```python
from build123d import *

# Parameters (mm, degrees)
SKETCH1_W                    = 119
SKETCH1_H                    = 89
BOSS_EXTRUDE2_DEPTH          = 3
SKETCH3_W                    = 89
SKETCH3_H                    = 89
SKETCH3_W_2                  = 85
SKETCH3_H_2                  = 85
BOSS_EXTRUDE3_DEPTH          = 25
SKETCH4_W                    = 87
SKETCH4_H                    = 87
CUT_EXTRUDE1_DEPTH           = 2
SKETCH6_W                    = 8
SKETCH6_H                    = 8
BOSS_EXTRUDE4_DEPTH          = 2
SKETCH7_R                    = 2
CUT_EXTRUDE2_DEPTH           = 4.8
SKETCH8_W                    = 9
SKETCH8_H                    = 11
SKETCH8_W_2                  = 12
SKETCH8_W_3                  = 13
SKETCH8_H_2                  = 12
CUT_EXTRUDE3_DEPTH           = 2
SKETCH9_W                    = 13
SKETCH9_H                    = 11
CUT_EXTRUDE4_DEPTH           = 2
SKETCH10_R                   = 1.6
CUT_EXTRUDE5_DEPTH           = 3
SKETCH11_W                   = 7
SKETCH11_H                   = 25
CUT_EXTRUDE6_DEPTH           = 1
FILLET2_R                    = 2
CSK_FOR_M3_SFHCS1_AT_2_COUNT = 2
CSK_FOR_M3_SFHCS1_AT_2_PITCH = 69
CSK_FOR_M3_SFHCS1_AT_3_COUNT = 2
CSK_FOR_M3_SFHCS1_AT_3_PITCH = 124.807852317
CSK_FOR_M3_SFHCS1_AT_4_COUNT = 2
CSK_FOR_M3_SFHCS1_AT_4_PITCH = 104


with BuildPart() as part:
    # Sketch1 → Boss-Extrude2 (new body)
    with BuildSketch(Plane(origin=(0, 0, 0), x_dir=(1, 0, 0), z_dir=(0, 1, 0))):
        Rectangle(SKETCH1_W, SKETCH1_H)
    extrude(amount=BOSS_EXTRUDE2_DEPTH)

    # Sketch3 → Boss-Extrude3 (add)
    with BuildSketch(Plane(origin=(0, 3, 0), x_dir=(1, 0, 0), z_dir=(0, 1, 0))):
        Rectangle(SKETCH3_W, SKETCH3_H)
        Rectangle(SKETCH3_W_2, SKETCH3_H_2, mode=Mode.SUBTRACT)
    extrude(amount=BOSS_EXTRUDE3_DEPTH)

    # Sketch4 → Cut-Extrude1 (cut)
    with BuildSketch(Plane(origin=(0, 28, 0), x_dir=(1, 0, 0), z_dir=(0, 1, 0))):
        Rectangle(SKETCH4_W, SKETCH4_H)
    extrude(amount=-CUT_EXTRUDE1_DEPTH, mode=Mode.SUBTRACT)

    # Sketch6 → Boss-Extrude4 (add)
    with BuildSketch(Plane(origin=(0, 3, 0), x_dir=(1, 0, 0), z_dir=(0, 1, 0))):
        with Locations((-38.5, -38.5)):
            Rectangle(SKETCH6_W, SKETCH6_H)
        with Locations((-38.5, 38.5)):
            Rectangle(SKETCH6_W, SKETCH6_H)
        with Locations((38.5, 38.5)):
            Rectangle(SKETCH6_W, SKETCH6_H)
        with Locations((38.5, -38.5)):
            Rectangle(SKETCH6_W, SKETCH6_H)
    extrude(amount=BOSS_EXTRUDE4_DEPTH)

    # Sketch7 → Cut-Extrude2 (cut)
    with BuildSketch(Plane(origin=(0, 5, 0), x_dir=(1, 0, 0), z_dir=(0, 1, 0))):
        with Locations((-38.5, 38.5)):
            Circle(SKETCH7_R)
        with Locations((38.5, 38.5)):
            Circle(SKETCH7_R)
        with Locations((-38.5, -38.5)):
            Circle(SKETCH7_R)
        with Locations((38.5, -38.5)):
            Circle(SKETCH7_R)
    extrude(amount=-CUT_EXTRUDE2_DEPTH, mode=Mode.SUBTRACT)

    # Sketch8 → Cut-Extrude3 (cut)
    with BuildSketch(Plane(origin=(-42.5, 0, 0), x_dir=(0, 0, -1), z_dir=(1, 0, 0))):
        with Locations((16.4, 13.5)):
            Rectangle(SKETCH8_W, SKETCH8_H)
        with Locations((1.4, 13.5)):
            Rectangle(SKETCH8_W_2, SKETCH8_H)
        with Locations((-14.5, 14)):
            Rectangle(SKETCH8_W_3, SKETCH8_H_2)
    extrude(amount=-CUT_EXTRUDE3_DEPTH, mode=Mode.SUBTRACT)

    # Sketch9 → Cut-Extrude4 (cut)
    with BuildSketch(Plane(origin=(0, 0, 42.5), x_dir=(-1, 0, 0), z_dir=(0, 0, -1))):
        with Locations((8.5, 13.5)):
            Rectangle(SKETCH9_W, SKETCH9_H)
        with Locations((25.5, 13.5)):
            Rectangle(SKETCH9_W, SKETCH9_H)
        with Locations((-8.5, 13.5)):
            Rectangle(SKETCH9_W, SKETCH9_H)
        with Locations((-25.5, 13.5)):
            Rectangle(SKETCH9_W, SKETCH9_H)
    extrude(amount=-CUT_EXTRUDE4_DEPTH, mode=Mode.SUBTRACT)

    # Sketch10 → Cut-Extrude5 (cut)
    with BuildSketch(Plane(origin=(0, 3, 0), x_dir=(1, 0, 0), z_dir=(0, 1, 0))):
        with Locations((-52, 34.5)):
            Circle(SKETCH10_R)
        with Locations((-52, -34.5)):
            Circle(SKETCH10_R)
        with Locations((52, 34.5)):
            Circle(SKETCH10_R)
        with Locations((52, -34.5)):
            Circle(SKETCH10_R)
    extrude(amount=-CUT_EXTRUDE5_DEPTH, mode=Mode.SUBTRACT)

    # Sketch11 → Cut-Extrude6 (cut)
    with BuildSketch(Plane(origin=(0, 3, 0), x_dir=(1, 0, 0), z_dir=(0, 1, 0))):
        with Locations((52, -14.77145541)):
            Rectangle(SKETCH11_W, SKETCH11_H)
    extrude(amount=-CUT_EXTRUDE6_DEPTH, mode=Mode.SUBTRACT)

    # Fillet2
    fillet2_edges = [part.edges().sort_by_distance(p)[0] for p in [
        (59.5, 3, 0),
        (52, 3, 44.5),
        (-52, 3, -44.5),
        (52, 3, -44.5),
        (-44.5, 3, 0),
        (-44.5, 15.5, -44.5),
        (-44.5, 15.5, 44.5),
        (44.5, 3, 0),
        (44.5, 15.5, 44.5),
        (44.5, 15.5, -44.5),
        (-59.5, 3, 0),
        (-59.5, 1.5, -44.5),
        (59.5, 1.5, -44.5),
        (59.5, 1.5, 44.5),
        (-59.5, 1.5, 44.5),
        (-52, 3, 44.5),
    ]]
    fillet(fillet2_edges, radius=FILLET2_R)

    # Sketch13 → CSK for M3 SFHCS1 (revolve, cut)
    with BuildSketch(Plane(origin=(52, 3, -34.5), x_dir=(0, 0, 1), z_dir=(1, 0, 0))):
        Polygon((0, 0), (0, 3), (1.7, 3), (1.7, 1.66), (3.36, 0), align=None)
    csk_for_m3_sfhcs1 = revolve(axis=Axis((52, 9.35, -34.5), (0, -1, 0)), mode=Mode.SUBTRACT)

    # CSK for M3 SFHCS1 at 2: CSK for M3 SFHCS1 ×2
    with Locations(*[(0, 0, i * CSK_FOR_M3_SFHCS1_AT_2_PITCH) for i in range(1, CSK_FOR_M3_SFHCS1_AT_2_COUNT)]):
        add(csk_for_m3_sfhcs1, mode=Mode.SUBTRACT)

    # CSK for M3 SFHCS1 at 3: CSK for M3 SFHCS1 ×2
    with Locations(*[Vector(-0.833280904, 0, 0.552849831) * (i * CSK_FOR_M3_SFHCS1_AT_3_PITCH) for i in range(1, CSK_FOR_M3_SFHCS1_AT_3_COUNT)]):
        add(csk_for_m3_sfhcs1, mode=Mode.SUBTRACT)

    # CSK for M3 SFHCS1 at 4: CSK for M3 SFHCS1 ×2
    with Locations(*[(-i * CSK_FOR_M3_SFHCS1_AT_4_PITCH, 0, 0) for i in range(1, CSK_FOR_M3_SFHCS1_AT_4_COUNT)]):
        add(csk_for_m3_sfhcs1, mode=Mode.SUBTRACT)


solid = part.part
```
Geometry check sheet. Reference: the model listing, model coordinates, mm. A direction names the side the tool comes from. Give positions to 0.01 mm unless a question says otherwise; leave off trailing zeros. Order: outer loops, then holes, each group sorted by start corner. A loop starts at its lowest first (then second) coordinate and runs counter-clockwise, first axis right, second up. Notation, with made-up numbers: (8, 75) - (59, 75) arc R37 ccw to (59, 112) - close; hole circle Ø2 at (-28.75, -37.5). An arc over 180 degrees is marked (long way). Write item = value, one per line. Start each with the question number.
1) Section check A-A (z = 17). Enter the section's corners in (x, y).
2) Section check D-D (y = 16.75). Count the separate pieces of the cut face and the enclosed holes in it, then the cut area to 3 significant figures.
3) Gauge pin test, flat ends, axial feed: pin 1 Ø12 at (y, z) = (25, 6.5) entering from +X; pin 2 Ø4 at (y, z) = (16, 20.5) entering from -X; pin 3 Ø1 at (x, y) = (-44, 13.5) entering from -Z. Record the tip position at first contact, or that the pin passes through.
4) Section check B-B (x = 52). Enter the section's corners in (y, z).
5) Draft check along X on faces 1 (the cylindrical face through (-38.934, 2.634, 40.452)), 2 (the flat face through (52, 3, -1)), 3 (the flat face through (44.5, 16, 1)). Enter one of: released by +X, released by -X, zero draft, split by the parting line, or undercut.
6) Scan lines: L1, parallel to Z at x = 52, y = 0.9; L2, parallel to Z at x = -38.5, y = 2.7; L3, parallel to X at y = 0.6, z = -34.5. Record each from-to range of solid material in increasing order.
7) Access from +Z, -Z, +X, -X, +Y, -Y to the whole of each face (thin tool, end or side, straight path). Record for faces 4 (the flat face through (-1, 14, -44.5)), 5 (the flat face through (-52, 3, -1)), 6 (the flat face through (36.7, 5, 36.7)).
8) Section check C-C (x = -38.5). Enter the section's corners in (y, z).
Geometry check:
q1.outline = (-59.5, 0) - (59.5, 0) - (59.5, 1) arc R2 ccw to (57.5, 3) - (55.5, 3) - (55.5, 2) - (48.5, 2) - (48.5, 3) - (46.5, 3) arc R2 cw to (44.5, 5) - (44.5, 28) - (43.5, 28) - (43.5, 26) - (42.5, 26) - (42.5, 3) - (-42.5, 3) - (-42.5, 8) - (-44.5, 8) - (-44.5, 5) arc R2 cw to (-46.5, 3) - (-57.5, 3) arc R2 ccw to (-59.5, 1) - close; (-44.5, 20) - (-42.5, 20) - (-42.5, 26) - (-43.5, 26) - (-43.5, 28) - (-44.5, 28) - close
q2.separate_pieces = 7
q2.enclosed_holes = 0
q2.area = 521 mm2
q3.pin_1 = 44.5
q3.pin_2 = -44.5
q3.pin_3 = -44.23
q4.outline = (0, -44.5) - (1, -44.5) arc R2 ccw to (3, -42.5) - (3, -37.86) - (1.34, -36.2) - (0, -36.2) - close; (0, -32.8) - (1.34, -32.8) - (3, -31.14) - (3, 2.27) - (2, 2.27) - (2, 27.27) - (3, 27.27) - (3, 31.14) - (1.34, 32.8) - (0, 32.8) - close; (0, 36.2) - (1.34, 36.2) - (3, 37.86) - (3, 42.5) arc R2 ccw to (1, 44.5) - (0, 44.5) - close
q5.face_1 = undercut
q5.face_2 = zero draft
q5.face_3 = released by +X
q6.L1 = -44.5 to -36.2, -32.8 to 32.8, 36.2 to 44.5
q6.L2 = -44.5 to -40.5, -36.5 to 36.5, 40.5 to 44.5
q6.L3 = -59.5 to -53.7, -50.3 to 50.3, 53.7 to 59.5
q7.face_4 = -Z, +X, -X, +Y, -Y
q7.face_5 = +Z, -Z, -X, +Y
q7.face_6 = +Y
q8.outline = (0, -44.5) - (28, -44.5) - (28, -43.5) - (26, -43.5) - (26, -42.5) - (5, -42.5) - (5, -40.5) - (0.2, -40.5) - (0.2, -36.5) - (5, -36.5) - (5, -34.5) - (3, -34.5) - (3, 34.5) - (5, 34.5) - (5, 36.5) - (0.2, 36.5) - (0.2, 40.5) - (5, 40.5) - (5, 42.5) - (26, 42.5) - (26, 43.5) - (28, 43.5) - (28, 44.5) - (0, 44.5) - close
